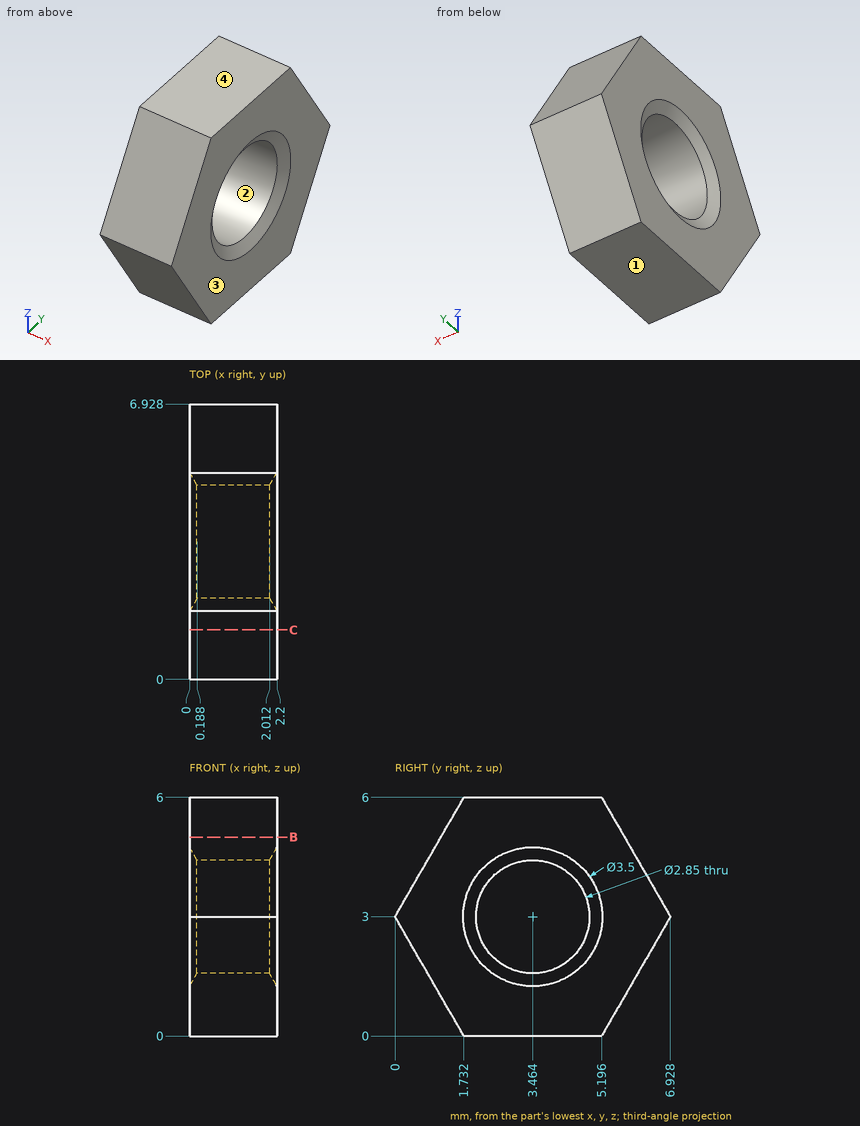
Job drawing, mm, ordinate dimensions from the low corner. One solid piece. Give positions to 0.01 mm unless a question says otherwise; leave off trailing zeros. Loops run counter-clockwise (first coordinate to the right, second up) from the corner with the lowest first, then second, coordinate; pieces in that order, holes last.
Item 1: Pull direction Z, two halves, no side cores. Call the marked faces 1, 2, 3 and 4: released by +Z, released by -Z, zero draft, split by the parting line, or undercut.
Answers follow:
face 1: released by -Z
face 2: undercut
face 3: zero draft
face 4: released by +Z
Item 2: Slice it at C-C, the plane y = 1.25. List the corners of the cut face in (x, z) (1 decimal).
Answers follow:
outline: (0, 0.8) - (2.2, 0.8) - (2.2, 5.2) - (0, 5.2) - close
Item 3: Drill centre lines: line 1 (Z direction, x = 1.75, y = 3.5) (1 decimal); line 2 (Z direction, x = 2.05, y = 3.75) (1 decimal); line 3 (X direction, y = 2, z = 2.25). Where is each one in solid material? Low to high.
Answers follow:
line 1: z = 0 to 1.6, 4.4 to 6
line 2: z = 0 to 1.5, 4.5 to 6
line 3: x = 0.06 to 2.14
Item 4: Slice it at B-B, the plane z = 5. List the corners of the cut face in (x, y) (1 decimal).
Answers follow:
outline: (0, 1.2) - (2.2, 1.2) - (2.2, 5.8) - (0, 5.8) - close
